Input: part model. Units: mm. Frame: model coordinates. A direction names the side the tool comes from. Round coordinates to 2 decimals unless told otherwise and drop trailing zeros. Order: outer loops, then holes, each group sorted by start corner. A loop starts at its lowest first (then second) coordinate and runs counter-clockwise, first axis right, second up. Notation, with made-up numbers: (-38.75, 32.25) -> (-17.75, 32.25) arc R28 cw to (-17.75, 59.25) -> close; hole circle Ø8 at (13.25, -37.5). An arc over 180 degrees is marked (long way). Use a Markdown table: item, result.
from build123d import *

# Parameters (mm, degrees)
SKETCH1_R               = 2.05
BOSS_EXTRUDE1_DEPTH     = 2
SKETCH2_R               = 3.87
BOSS_EXTRUDE2_DEPTH     = 10
SKETCH4_R               = 3
BOSS_EXTRUDE3_DEPTH     = 1
CUT_EXTRUDE2_DEPTH      = 15
CUT_EXTRUDE3_DEPTH      = 22.231780641
CUT_EXTRUDE3_DEPTH_BACK = 22.231780641
SKETCH9_R               = 1
CHAMFER1_SIZE           = 0.2


with BuildPart() as part:
    # Sketch1 → Boss-Extrude1 (new body)
    with BuildSketch(Plane(origin=(0, 0, 0), x_dir=(1, 0, 0), z_dir=(0, 1, 0))):
        with BuildLine():
            Line((-9.06012954, 6.238112913), (-9.06012954, -6.238112913))
            ThreePointArc((-9.06012954, -6.238112913), (-0.104590041, -10.999502758), (8.93987046, -6.40926799))
            Line((8.93987046, -6.40926799), (8.93987046, 6.40926799))
            ThreePointArc((8.93987046, 6.40926799), (-0.104590041, 10.999502758), (-9.06012954, 6.238112913))
        make_face()
        with Locations(Location((-4.917973081, 4.788086362, 0), (0, 0, 270))):
            Circle(SKETCH1_R, mode=Mode.SUBTRACT)
        with Locations(Location((4.788086362, 4.917973081, 0), (0, 0, 270))):
            Circle(SKETCH1_R, mode=Mode.SUBTRACT)
        with Locations(Location((4.917973081, -4.788086362, 0), (0, 0, 270))):
            Circle(SKETCH1_R, mode=Mode.SUBTRACT)
        with Locations(Location((-4.788086362, -4.917973081, 0), (0, 0, 270))):
            Circle(SKETCH1_R, mode=Mode.SUBTRACT)
    extrude(amount=BOSS_EXTRUDE1_DEPTH)

    # Sketch2 → Boss-Extrude2 (add)
    with BuildSketch(Plane(origin=(0, 2, 0), x_dir=(1, 0, 0), z_dir=(0, 1, 0))):
        with Locations(Location((0, 0, 0), (0, 0, 270))):
            Circle(SKETCH2_R)
    extrude(amount=BOSS_EXTRUDE2_DEPTH)

    # Sketch3 → Revolve1 (revolve)
    with BuildSketch(Plane.XY):
        with BuildLine():
            Line((0, 15.87), (0, 12))
            Line((0, 12), (3.87, 12))
            ThreePointArc((3.87, 12), (2.736503243, 14.736503243), (0, 15.87))
        make_face()
    revolve(axis=Axis((0, 15.87, 0), (0, -1, 0)))

    # Sketch4 → Boss-Extrude3 (add)
    with BuildSketch(Plane.XZ):
        with Locations(Location((0, 0, 0), (0, 0, 270))):
            Circle(SKETCH4_R)
    extrude(amount=BOSS_EXTRUDE3_DEPTH)

    # Sketch7 → Cut-Extrude2 (cut)
    with BuildSketch(Plane(origin=(0, 20, 0), x_dir=(1, 0, 0), z_dir=(0, 1, 0))):
        with BuildLine():
            Line((-7.332454233, 1), (7.579147316, 1))
            ThreePointArc((7.579147316, 1), (8.579147316, 0), (7.579147316, -1))
            Line((7.579147316, -1), (-7.332454233, -1))
            ThreePointArc((-7.332454233, -1), (-8.332454233, 0), (-7.332454233, 1))
        make_face()
    extrude(amount=-CUT_EXTRUDE2_DEPTH, mode=Mode.SUBTRACT)

    # Sketch9 → Cut-Extrude3 (cut, two sides: drawn at the far end of the back side and taken through both)
    with BuildSketch(Plane.XY.offset(-CUT_EXTRUDE3_DEPTH_BACK)):
        with Locations((0, 10.5)):
            Circle(SKETCH9_R)
    extrude(amount=CUT_EXTRUDE3_DEPTH + CUT_EXTRUDE3_DEPTH_BACK, mode=Mode.SUBTRACT)

    # Chamfer1
    chamfer1_edges = [part.edges().sort_by_distance(p)[0] for p in [
        (-4.917973081, 2, -6.838086362),
        (-0.104590041, 2, 10.999502758),
        (4.788086362, 2, -6.967973081),
        (8.93987046, 2, 0),
        (4.917973081, 2, 2.738086362),
        (-4.788086362, 2, 2.867973081),
        (0, 2, -3.87),
        (-0.104590041, 2, -10.999502758),
        (-9.06012954, 2, 0),
    ]]
    chamfer(chamfer1_edges, length=CHAMFER1_SIZE)


solid = part.part
1) Cut plane D-D on z = 0. Return loops of the section in (x, y), and give its area (3 significant figures).
Results found:
| item | result |
|---|---|
| outline | (-9.06, 0) -> (-3, 0) -> (-3, -1) -> (3, -1) -> (3, 0) -> (8.94, 0) -> (8.94, 1.8) -> (8.74, 2) -> (4.07, 2) -> (3.87, 2.2) -> (3.87, 5) -> (-3.87, 5) -> (-3.87, 2.2) -> (-4.07, 2) -> (-8.86, 2) -> (-9.06, 1.8) -> close |
| area | 65.2 mm² |
2) Line query: L1, parallel to Y at x = -6.75, z = 6.25; L2, parallel to Y at x = 0.75, z = -2.25; L3, parallel to Y at x = -0.5, z = 1.5. Output: solid intervals per line, ascending. Write a range as [from, to].
Results found:
| item | result |
|---|---|
| L1 | y = [0, 2] |
| L2 | y = [-1, 9.84], [11.16, 15.06] |
| L3 | y = [-1, 9.63], [11.37, 15.53] |
3) Set-up query: faces 4 (the flat face through (2, 0, -3)), 5 (the flat face through (0, 9, -1)), 6 (the flat face through (0, -1, 0)), 7 (the cylindrical face through (1.16, 7.03, 3.69)), 8 (the flat face through (-9.06, 1, 0)). Return all of +Z, -Z, +X, -X, +Y, -Y with unobstructed straight access to the full face (end or side cutting, diameter ignored); none if empty.
Results found:
| item | result |
|---|---|
| face 4 | -Y |
| face 5 | +X, -X, +Y |
| face 6 | +Z, -Z, +X, -X, -Y |
| face 7 | +Y |
| face 8 | +Z, -Z, -X, +Y, -Y |
4) Pull-direction query (X, two-part tool) for faces 1 (the flat face through (8.94, 1, 0)), 2 (the cylindrical face through (3.67, 0.89, 3.16)), 3 (the flat face through (0, 9, 1)); classes: +X half, -X half, draft (parallel to the pull), parting line (faces both ways), or undercut.
Results found:
| item | result |
|---|---|
| face 1 | +X half |
| face 2 | undercut |
| face 3 | draft |
5) Cut plane A-A on x = 0. Return loops of the section in (y, z), and give its area (3 significant figures).
Results found:
| item | result |
|---|---|
| outline | (-1, -3) -> (0, -3) -> (0, -11) -> (1.8, -11) -> (2, -10.8) -> (2, -4.07) -> (2.2, -3.87) -> (9.5, -3.87) -> (9.5, -1) -> (5, -1) -> (5, 1) -> (9.5, 1) -> (9.5, 3.87) -> (2.2, 3.87) -> (2, 4.07) -> (2, 10.8) -> (1.8, 11) -> (0, 11) -> (0, 3) -> (-1, 3) -> close; (11.5, -3.87) -> (12, -3.87) arc R3.87 ccw to (15.74, -1) -> (11.5, -1) -> close; (11.5, 1) -> (15.74, 1) arc R3.87 ccw to (12, 3.87) -> (11.5, 3.87) -> close |
| area | 118 mm² |
6) Cut plane B-B on y = 10.5. Return loops of the section in (x, z), and give its area (3 significant figures).
Results found:
| item | result |
|---|---|
| outline | (-3.74, -1) arc R3.87 ccw to (-1, -3.74) -> (-1, -1) -> close; (-3.74, 1) -> (-1, 1) -> (-1, 3.74) arc R3.87 ccw to start; (1, -3.74) arc R3.87 ccw to (3.74, -1) -> (1, -1) -> close; (1, 1) -> (3.74, 1) arc R3.87 ccw to (1, 3.74) -> close |
| area | 20.4 mm² |
7) Cut plane C-C on y = 6. Return loops of the section in (x, z).
Results found:
| item | result |
|---|---|
| outline | (-3.74, -1) arc R3.87 ccw to (3.74, -1) -> close; (-3.74, 1) -> (3.74, 1) arc R3.87 ccw to start |
8) Pin query (flat end, axial travel): pin 1 Ø8 at (x, y) = (-6.5, 9) entering from -Z; pin 2 Ø1 at (x, z) = (-1, 0) entering from +Y; pin 3 Ø5.5 at (x, z) = (-4.79, 4.92) entering from +Y; pin 4 Ø5.5 at (x, z) = (-4.5, 3.5) entering from -Y. Return the tip coordinate at first contact, or that it passes through.
Results found:
| item | result |
|---|---|
| pin 1 | stops at z = -2.95 |
| pin 2 | stops at y = 5 |
| pin 3 | stops at y = 2 |
| pin 4 | stops at y = -1 |
